Source: CAD feature listing. Evaluate the final solid. Frame: model axes, mm. A direction names the side the tool comes from. Round coordinates to 2 decimals unless told otherwise and drop trailing zeros. Order: outer loops, then holes, each group sorted by start corner. A loop starts at its lowest first (then second) coordinate and runs counter-clockwise, first axis right, second up. Notation, with made-up numbers: (14, -29) -> (36, -29) arc R23 ccw to (36, 2) -> close; hole circle Ø8 at (41, 33). An arc over 180 degrees is marked (long way). One line per item, written item: value. Start each with the question number.
1) Reachability of faces 4 (the face through (57, 44.5, 5)), 5 (the face through (-43, -1, 5)), 6 (the face through (-47, 86, 5)) from +Z, -Z, +X, -X, +Y, -Y: full face, straight path, thin tool, end or side. Return the list, or none.
2) Pin query (flat end, axial travel): P1, Ø3, axis at x = 36.5, y = 47.5, coming from the +Z side; P2, Ø5, axis at y = -8, z = 3, coming from the +X side; P3, Ø3, axis at y = 82.5, z = 4, coming from the -X side; P4, Ø4, axis at x = -50.5, y = 45.5, coming from the +Z side. Return the tip coordinate at first contact, or that it passes through.
3) Section B-B (x = -54.5). Return the cut outline in (y, z).
4) Section A-A (y = 78). Return the cut outline in (x, z).
5) Section C-C (z = 3.25). State how many separate pieces and enclosed holes the cut face has, and give its area (3 significant figures).
6) Ray query, L1, parallel to Y at x = -15.5, z = 5.5; L2, parallel to X at y = 70, z = 5.5; L3, parallel to Y at x = -49, z = 0.75. Return the intervals inside material, ascending.
7) Mould query, pull axis X, two halves, no side actions, for faces 1 (the face through (-1, 44.5, 5)), 2 (the face through (57, -40.5, 5)), 3 (the face through (-47, 1, 5)). Classes: pulls with the +X half, pulls with the -X half, needs draft (parallel to the pull), parting line crosses it, or undercut.
```python
from build123d import *

# Parameters (mm, degrees)
SKETCH1_W           = 86
SKETCH1_H           = 81
BOSS_EXTRUDE1_DEPTH = 10
FILLET1_R           = 3


with BuildPart() as part:
    # Sketch1 → Boss-Extrude1 (new body)
    with BuildSketch(Plane.XY):
        Polygon((-64, 129.5), (-64, 125.5), (-47, 125.5), (-47, 44.5), (-64, 44.5), (-64, 40.5), (-47, 40.5), (-47, -40.5), (-64, -40.5), (-64, -44.5), (0, -44.5), (64, -44.5), (64, -40.5), (47, -40.5), (47, 40.5), (64, 40.5), (64, 44.5), (47, 44.5), (47, 125.5), (64, 125.5), (64, 129.5), (0, 129.5), align=None)
        Rectangle(SKETCH1_W, SKETCH1_H, mode=Mode.SUBTRACT)
        with Locations((0, 85)):
            Rectangle(SKETCH1_W, SKETCH1_H, mode=Mode.SUBTRACT)
    extrude(amount=BOSS_EXTRUDE1_DEPTH)

    # Fillet1
    fillet1_edges = [part.edges().sort_by_distance(p)[0] for p in [
        (-43, -40.5, 5),
        (43, -40.5, 5),
        (43, 40.5, 5),
        (-43, 40.5, 5),
        (-47, 44.5, 5),
        (-47, 125.5, 5),
        (47, 125.5, 5),
        (47, 44.5, 5),
        (47, 40.5, 5),
        (47, -40.5, 5),
        (-47, -40.5, 5),
        (-47, 40.5, 5),
        (43, 44.5, 5),
        (43, 125.5, 5),
        (-43, 125.5, 5),
        (-43, 44.5, 5),
    ]]
    fillet(fillet1_edges, radius=FILLET1_R)


solid = part.part
```
Findings:
1. face 4: +Z, -Z, +X
1. face 5: +Z, -Z
1. face 6: +Z, -Z, -X
2. P1: through
2. P2: x = 47
2. P3: x = -47
2. P4: z = 10
3. outline: (-44.5, 0) -> (-40.5, 0) -> (-40.5, 10) -> (-44.5, 10) -> close; (40.5, 0) -> (44.5, 0) -> (44.5, 10) -> (40.5, 10) -> close; (125.5, 0) -> (129.5, 0) -> (129.5, 10) -> (125.5, 10) -> close
4. outline: (-47, 0) -> (-43, 0) -> (-43, 10) -> (-47, 10) -> close; (43, 0) -> (47, 0) -> (47, 10) -> (43, 10) -> close
5. separate pieces: 1
5. enclosed holes: 2
5. area: 2,860 mm2
6. L1: -44.5 to -40.5, 40.5 to 44.5, 125.5 to 129.5
6. L2: -47 to -43, 43 to 47
6. L3: -44.5 to -40.33, 40.33 to 44.67, 125.33 to 129.5
7. face 1: undercut
7. face 2: needs draft
7. face 3: pulls with the -X half
